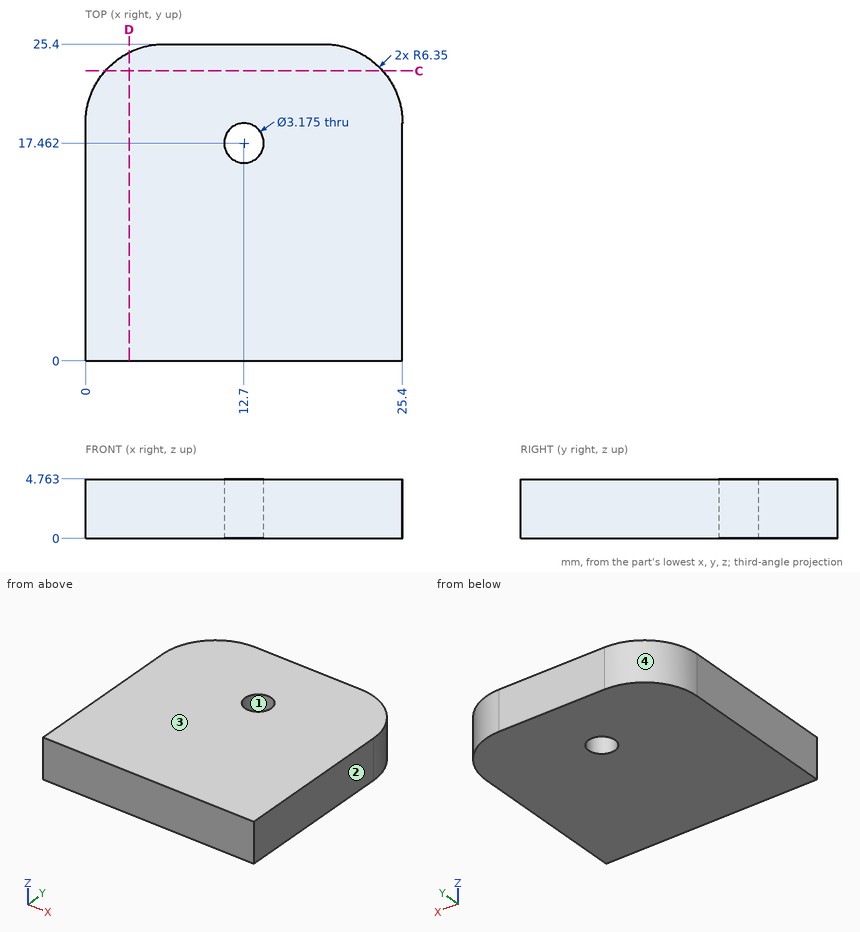
Input: dimensioned drawing with shaded views. Units: mm. Origin: part minimum x, y, z. Round coordinates to 2 decimals unless told otherwise and drop trailing zeros. Order: outer loops, then holes, each group sorted by start corner. A loop starts at its lowest first (then second) coordinate and runs counter-clockwise, first axis right, second up. Notation, with made-up numbers: (-15, -23) - (22, -23) arc R28 ccw to (22, 14) - close; hole circle Ø2 at (66.25, 8.5). An arc over 180 degrees is marked (long way). Answer as a JSON object with one key per item and string values. Group by question number.
(1) Cut plane D-D (x = 3.5). Return loops of the section in (y, z) (1 decimal).
(2) Cut plane C-C (y = 23.25). Return loops of the section in (x, z).
(3) Material intervals for probe 1 along X at (y, z) = (16.75, 4); probe 2 along Y at (x, z) = (12, 2.5); probe 3 along Y at (x, z) = (21.5, 1.35), sorted ascending. Write a range as from..to.
(4) Draft query along X for the marked faces 1, 2, 3 and 4. Return one class per face: released by +X, released by -X, zero draft, split by the parting line, or undercut.
Here are the results:
{
 "1": {"outline": "(0, 0) - (24.7, 0) - (24.7, 4.8) - (0, 4.8) - close"},
 "2": {"outline": "(1.59, 0) - (23.81, 0) - (23.81, 4.76) - (1.59, 4.76) - close"},
 "3": {"probe 1": "x = 0..11.28, 14.12..25.4", "probe 2": "y = 0..16.04, 18.89..25.4", "probe 3": "y = 0..24.91"},
 "4": {"face 1": "undercut", "face 2": "released by +X", "face 3": "zero draft", "face 4": "released by -X"}
}
